The model under review builds one solid part; all positions refer to its coordinate system, in mm. Give positions to 0.01 mm unless a question says otherwise; leave off trailing zeros. Loops run counter-clockwise (first coordinate to the right, second up) from the corner with the lowest first, then second, coordinate; pieces in that order, holes last. Notation, with made-up numbers: M -31.5,13 L -14.5,13 A22 cw -14.5,44 Z; hole C -18.75,72 d3. An arc over 180 degrees is marked long. Return JSON: item names as keys, results as strings.
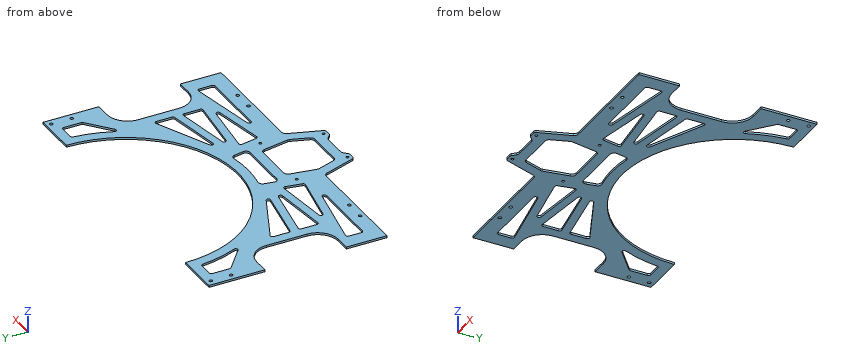
```python
from build123d import *

# Parameters (mm, degrees)
SKETCH_1_W              = 306
SKETCH_1_H              = 175
EXTRUDE_1_DEPTH         = 2
SKETCH_2_R              = 110
SKETCH_2_W              = 35
SKETCH_2_H              = 80
CUT_EXTRUDE_1_DEPTH     = 177.264715698
FILLET_1_R              = 20
HOLE_WIZARD_3_2_3_2_1_D = 3.2
SKETCH_5_W              = 76
SKETCH_5_H              = 35
EXTRUDE_2_DEPTH         = 2
HOLE_WIZARD_2_6_2_6_1_D = 2.6
CUT_EXTRUDE_2_DEPTH     = 197.008290641
FILLET_2_R              = 2
FILLET_3_R              = 4
CUT_EXTRUDE_3_DEPTH     = 197.008290641
FILLET_4_R              = 2
FILLET_4_OF_MIRROR_2_R  = 2
CUT_EXTRUDE_4_DEPTH     = 197.008290641
FILLET_5_R              = 4
HOLE_WIZARD_3_2_3_2_2_D = 3.2
CUT_EXTRUDE_5_DEPTH     = 197.008290641
FILLET_7_R              = 2
FILLET_7_OF_MIRROR_4_R  = 2


with BuildPart() as part:
    # 草图1 → 凸台-拉伸1 (new body)
    with BuildSketch(Plane.XY):
        Rectangle(SKETCH_1_W, SKETCH_1_H)
    extrude(amount=EXTRUDE_1_DEPTH)

    # 草图2 → 切除-拉伸1 (cut, through all)
    with BuildSketch(Plane.XY.offset(2)):
        with Locations((0, 87.5)):
            Circle(SKETCH_2_R)
        with Locations((-135.5, -7.5)):
            Rectangle(SKETCH_2_W, SKETCH_2_H)
        with Locations((135.5, -7.5)):
            Rectangle(SKETCH_2_W, SKETCH_2_H)
    extrude(amount=-CUT_EXTRUDE_1_DEPTH, mode=Mode.SUBTRACT)

    # 圆角1
    fillet_1_edges = [part.edges().sort_by_distance(p)[0] for p in [
        (118, -47.5, 1),
        (118, 32.5, 1),
        (-118, 32.5, 1),
        (-118, -47.5, 1),
    ]]
    fillet(fillet_1_edges, radius=FILLET_1_R)

    # Ø3.2 (3.2) 直径孔1 (through all)
    with Locations(Plane(origin=(113, -82.5, 2), x_dir=(1, 0, 0), z_dir=(0, 0, 1))):
        with Locations((0, 0), (-20, 0)):
            hole_wizard_3_2_3_2_1 = Hole(HOLE_WIZARD_3_2_3_2_1_D / 2)

    # 镜向1: Ø3.2 (3.2) 直径孔1 across plane
    add(hole_wizard_3_2_3_2_1.mirror(Plane(origin=(0, 0, 0), x_dir=(0, 0, 1), z_dir=(1, 0, 0))), mode=Mode.SUBTRACT)

    # 草图5 → 凸台-拉伸2 (add)
    with BuildSketch(Plane.XY.offset(2)):
        with Locations((0, -105)):
            Rectangle(SKETCH_5_W, SKETCH_5_H)
    extrude(amount=-EXTRUDE_2_DEPTH)

    # Ø2.6 (2.6) 直径孔1 (through all)
    with Locations(Plane(origin=(-33.75, -62.5, 2), x_dir=(1, 0, 0), z_dir=(0, 0, 1))):
        with Locations((0, 0), (67.5, 0), (11.75, -56), (55.75, -56)):
            Hole(HOLE_WIZARD_2_6_2_6_1_D / 2)

    # 草图8 → 切除-拉伸2 (cut, through all)
    with BuildSketch(Plane.XY.offset(2)):
        Polygon((38, -122.5), (26, -122.5), (38, -87.5), align=None)
        Polygon((-38, -87.5), (-26, -122.5), (-38, -122.5), align=None)
        Polygon((-18, -122.5), (-13, -117.5), (13, -117.5), (18, -122.5), align=None)
    extrude(amount=-CUT_EXTRUDE_2_DEPTH, mode=Mode.SUBTRACT)

    # 圆角2
    fillet_2_edges = [part.edges().sort_by_distance(p)[0] for p in [
        (26, -122.5, 1),
        (-26, -122.5, 1),
        (18, -122.5, 1),
        (-18, -122.5, 1),
    ]]
    fillet(fillet_2_edges, radius=FILLET_2_R)

    # 圆角3
    fillet_3_edges = [part.edges().sort_by_distance(p)[0] for p in [
        (-38, -87.5, 1),
        (38, -87.5, 1),
        (-13, -117.5, 1),
        (13, -117.5, 1),
    ]]
    fillet(fillet_3_edges, radius=FILLET_3_R)

    # 草图9 → 切除-拉伸3 (cut, through all)
    with BuildSketch(Plane.XY.offset(2)):
        Polygon((-138, -55.5), (-138, -72.5), (-48, -72.5), align=None)
        with BuildLine():
            Line((-21.498069498, -104.797297297), (-27.279305729, -87.93535829))
            ThreePointArc((-27.279305729, -87.93535829), (-27.483396797, -86.949275011), (-27.434752957, -85.943468283))
            Line((-27.434752957, -85.943468283), (-23.002234561, -60.805407289))
            ThreePointArc((-23.002234561, -60.805407289), (-21.634153988, -58.435822228), (-19.063003549, -57.5))
            Line((-19.063003549, -57.5), (19.063003549, -57.5))
            ThreePointArc((19.063003549, -57.5), (21.634153988, -58.435822228), (23.002234561, -60.805407289))
            Line((23.002234561, -60.805407289), (27.434752957, -85.943468283))
            ThreePointArc((27.434752957, -85.943468283), (27.483396797, -86.949275011), (27.279305729, -87.93535829))
            Line((27.279305729, -87.93535829), (21.498069498, -104.797297297))
            ThreePointArc((21.498069498, -104.797297297), (20.039238489, -106.754933885), (17.714285714, -107.5))
            Line((17.714285714, -107.5), (-17.714285714, -107.5))
            ThreePointArc((-17.714285714, -107.5), (-20.039238489, -106.754933885), (-21.498069498, -104.797297297))
        make_face()
        Polygon((-108, -53.025201394), (-43, -65.302979172), (-39.222222222, -45.302979172), align=None)
        Polygon((-108, -24.974934041), (-108, -44.974934041), (-38, -37.115483314), align=None)
        Polygon((-108, 3.144495264), (-108, -16.855504736), (-38, -28.996054009), align=None)
    cut_extrude_3 = extrude(amount=-CUT_EXTRUDE_3_DEPTH, mode=Mode.SUBTRACT)

    # 圆角4
    fillet_4_edges = [part.edges().sort_by_distance(p)[0] for p in [
        (-108, -24.974934041, 1),
        (-38, -37.115483314, 1),
        (-108, -44.974934041, 1),
        (-108, 3.144495264, 1),
        (-38, -28.996054009, 1),
        (-108, -16.855504736, 1),
        (-108, -53.025201394, 1),
        (-39.222222222, -45.302979172, 1),
        (-43, -65.302979172, 1),
        (-138, -55.5, 1),
        (-48, -72.5, 1),
        (-138, -72.5, 1),
    ]]
    fillet(fillet_4_edges, radius=FILLET_4_R)

    # 镜向2: 切除-拉伸3 across plane
    add(cut_extrude_3.mirror(Plane(origin=(0, 0, 0), x_dir=(0, 0, 1), z_dir=(1, 0, 0))), mode=Mode.SUBTRACT)

    # 圆角4 of 镜向2
    fillet_4_of_mirror_2_edges = [part.edges().sort_by_distance(p)[0] for p in [
        (108, -24.974934041, 1),
        (38, -37.115483314, 1),
        (108, -44.974934041, 1),
        (108, 3.144495264, 1),
        (38, -28.996054009, 1),
        (108, -16.855504736, 1),
        (108, -53.025201394, 1),
        (39.222222222, -45.302979172, 1),
        (43, -65.302979172, 1),
        (138, -55.5, 1),
        (48, -72.5, 1),
        (138, -72.5, 1),
    ]]
    fillet(fillet_4_of_mirror_2_edges, radius=FILLET_4_OF_MIRROR_2_R)

    # 草图10 → 切除-拉伸4 (cut, through all)
    with BuildSketch(Plane.XY.offset(2)):
        with BuildLine():
            Line((-29.460383454, -47.5), (-26.085046608, -29.630569637))
            ThreePointArc((-26.085046608, -29.630569637), (0, -32.5), (26.085046608, -29.630569637))
            Line((26.085046608, -29.630569637), (29.460383454, -47.5))
            Line((29.460383454, -47.5), (-29.460383454, -47.5))
        make_face()
    extrude(amount=-CUT_EXTRUDE_4_DEPTH, mode=Mode.SUBTRACT)

    # 圆角5
    fillet_5_edges = [part.edges().sort_by_distance(p)[0] for p in [
        (29.460383454, -47.5, 1),
        (-29.460383454, -47.5, 1),
        (-26.085046608, -29.630569637, 1),
        (26.085046608, -29.630569637, 1),
    ]]
    fillet(fillet_5_edges, radius=FILLET_5_R)

    # Ø3.2 (3.2) 直径孔2 (through all)
    with Locations(Plane(origin=(147, 82.5, 2), x_dir=(1, 0, 0), z_dir=(0, 0, 1))):
        with Locations((0, 0), (0, -20)):
            hole_wizard_3_2_3_2_2 = Hole(HOLE_WIZARD_3_2_3_2_2_D / 2)

    # 镜向3: Ø3.2 (3.2) 直径孔2 across plane
    add(hole_wizard_3_2_3_2_2.mirror(Plane(origin=(0, 0, 0), x_dir=(0, 0, 1), z_dir=(1, 0, 0))), mode=Mode.SUBTRACT)

    # 草图13 → 切除-拉伸5 (cut, through all)
    with BuildSketch(Plane.XY.offset(2)):
        with BuildLine():
            Line((-137, 77.5), (-119.582607431, 77.5))
            ThreePointArc((-119.582607431, 77.5), (-115.231385377, 54.007794577), (-106.312384413, 31.843222151))
            Line((-106.312384413, 31.843222151), (-137, 57.5))
            Line((-137, 57.5), (-137, 77.5))
        make_face()
    cut_extrude_5 = extrude(amount=-CUT_EXTRUDE_5_DEPTH, mode=Mode.SUBTRACT)

    # 圆角7
    fillet_7_edges = [part.edges().sort_by_distance(p)[0] for p in [
        (-137, 57.5, 1),
        (-137, 77.5, 1),
        (-119.582607431, 77.5, 1),
        (-106.312384413, 31.843222151, 1),
    ]]
    fillet(fillet_7_edges, radius=FILLET_7_R)

    # 镜向4: 切除-拉伸5 across plane
    add(cut_extrude_5.mirror(Plane(origin=(0, 0, 0), x_dir=(0, 0, 1), z_dir=(1, 0, 0))), mode=Mode.SUBTRACT)

    # 圆角7 of 镜向4
    fillet_7_of_mirror_4_edges = [part.edges().sort_by_distance(p)[0] for p in [
        (137, 57.5, 1),
        (137, 77.5, 1),
        (119.582607431, 77.5, 1),
        (106.312384413, 31.843222151, 1),
    ]]
    fillet(fillet_7_of_mirror_4_edges, radius=FILLET_7_OF_MIRROR_4_R)


solid = part.part
```
1) Insertion check: pin 1 (1 mm diameter, centred on y = -33.5, z = 0.5, fed in from -X); pin 2 (3.5 mm diameter, centred on x = 22, y = -118.5, fed in from +Z); pin 3 (0.6 mm diameter, centred on x = 86.5, z = 1, fed in from -Y); pin 4 (1 mm diameter, centred on x = 96, z = 0.5, fed in from +Y). Each pin has a flat end and moves straight along its axis. Give the tip position at first contact, or say it passes through.
From the geometry:
{"pin 1": "x = -119.09", "pin 2": "z = 2", "pin 3": "y = -87.5", "pin 4": "y = 34.7"}
2) Consider section B-B on y = 7.5. Write out the cut boundary in (x, z), then the cut area to 3 significant figures.
From the geometry:
{"outline": "M -118,0 L -75.5,0 L -75.5,2 L -118,2 Z; M 75.5,0 L 118,0 L 118,2 L 75.5,2 Z", "area": "170 mm²"}
3) Consider section D-D on z = 0.4. Count the separate pieces of the cut face and the enclosed holes in it, then the cut area to 3 significant figures.
From the geometry:
{"separate pieces": "1", "enclosed holes": "24", "area": "21,300 mm²"}
4) Consider section A-A on x = 0. Write out the cut boundary in (y, z), then the cut area to 3 significant figures.
From the geometry:
{"outline": "M -117.5,0 L -107.5,0 L -107.5,2 L -117.5,2 Z; M -57.5,0 L -47.5,0 L -47.5,2 L -57.5,2 Z; M -32.5,0 L -22.5,0 L -22.5,2 L -32.5,2 Z", "area": "60.0 mm²"}
5) Wall thickness on L1, parallel to Y at x = 147, z = 0.9; L2, parallel to X at y = -82.5, z = 1.3; L3, parallel to Y at x = 93, z = 1.4: over which ranges is each line inside the solid? List them lowest first. Write a range as from..to.
From the geometry:
{"L1": "-87.5..-47.5, 32.5..60.9, 64.1..80.9, 84.1..87.5", "L2": "-153..-114.6, -111.4..-94.6, -91.4..-26.83, 26.83..91.4, 94.6..111.4, 114.6..153", "L3": "-87.5..-84.1, -80.9..-72.5, -64..-55.86, -51.34..-43.29, -27.58..-19.46, -3.74..28.75"}
6) Consider section C-C on y = 50. Write out the cut boundary in (x, z), then the cut area to 3 significant figures.
From the geometry:
{"outline": "M -153,0 L -128.03,0 L -128.03,2 L -153,2 Z; M -113.99,0 L -103.41,0 L -103.41,2 L -113.99,2 Z; M 103.41,0 L 113.99,0 L 113.99,2 L 103.41,2 Z; M 128.03,0 L 153,0 L 153,2 L 128.03,2 Z", "area": "142 mm²"}
